from build123d import *

# Parameters (mm, degrees)
SKETCH1_W           = 22
SKETCH1_H           = 22
SKETCH1_W_2         = 20.1
SKETCH1_H_2         = 20.1
BOSS_EXTRUDE1_DEPTH = 15
SKETCH2_W           = 22
SKETCH2_H           = 22
BOSS_EXTRUDE2_DEPTH = 2


with BuildPart() as part:
    # Sketch1 → Boss-Extrude1 (new body)
    # profile 1 of 3: a face of its own
    with BuildSketch(Plane(origin=(0, 0, 0), x_dir=(1, 0, 0), z_dir=(0, 1, 0))):
        Rectangle(SKETCH1_W, SKETCH1_H)
        Rectangle(SKETCH1_W_2, SKETCH1_H_2, mode=Mode.SUBTRACT)
    # profile 2 of 3: a face of its own
    with BuildSketch(Plane(origin=(0, 0, 0), x_dir=(1, 0, 0), z_dir=(0, 1, 0))):
        Polygon((1.245, 10.05), (-1.245, 10.05), (-1.245, 8.05), (-5, 8.05), (-0.799132047, 5.15), (0.799132047, 5.15), (5, 8.05), (1.245, 8.05), align=None)
    # profile 3 of 3: a face of its own
    with BuildSketch(Plane(origin=(0, 0, 0), x_dir=(1, 0, 0), z_dir=(0, 1, 0))):
        Polygon((-1.245, -8.05), (-1.245, -10.05), (1.245, -10.05), (1.245, -8.05), (5, -8.05), (0.799132047, -5.15), (-0.799132047, -5.15), (-5, -8.05), align=None)
    extrude(amount=BOSS_EXTRUDE1_DEPTH)

    # Sketch2 → Boss-Extrude2 (add)
    with BuildSketch(Plane.XZ):
        Rectangle(SKETCH2_W, SKETCH2_H)
    extrude(amount=BOSS_EXTRUDE2_DEPTH)


solid = part.part
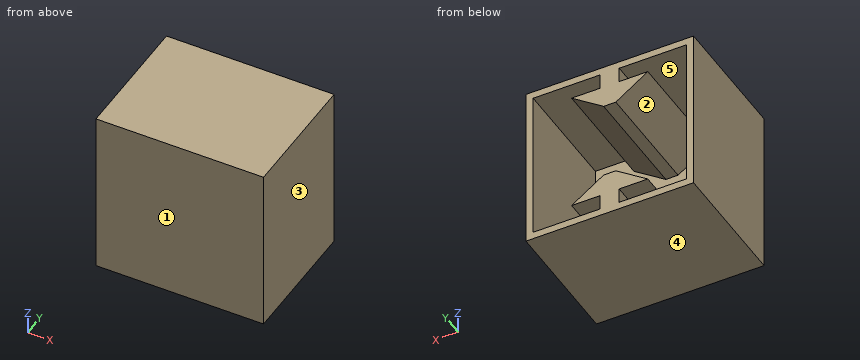
Model file for the job. Use its own axes, mm. Face numbers are marked on the shaded views. A direction names the side the tool comes from. Give positions to 0.01 mm unless a question says otherwise; leave off trailing zeros. Loops run counter-clockwise (first coordinate to the right, second up) from the corner with the lowest first, then second, coordinate; pieces in that order, holes last.
Item 1: Mould opens along X. For the marked faces 3, 4 and 5 say: +X half, -X half, draft (parallel to the pull), parting line (faces both ways), or undercut.
Check values:
face 3: +X half
face 4: draft
face 5: undercut
Item 2: Slice it at A-A (y = 6.5). Write the cut outline in (x, z) (3 decimals).
Check values:
outline: (-11, -11) - (11, -11) - (11, 11) - (-11, 11) - close; hole (-10.05, -10.05) - (-1.245, -10.05) - (-1.245, -8.05) - (-5, -8.05) - (-0.799, -5.15) - (0.799, -5.15) - (5, -8.05) - (1.245, -8.05) - (1.245, -10.05) - (10.05, -10.05) - (10.05, 10.05) - (1.245, 10.05) - (1.245, 8.05) - (5, 8.05) - (0.799, 5.15) - (-0.799, 5.15) - (-5, 8.05) - (-1.245, 8.05) - (-1.245, 10.05) - (-10.05, 10.05) - close
Item 3: Which spindle directions (+Z, -Z, +X, -X, +Y, -Y) get a long thin tool onto all of the face, cutting with end or side? Do the marked faces 1 and 2. Say none if no direction does.
Check values:
face 1: +Z, -Z, +X, -X, -Y
face 2: +Y
Item 4: Slice it at D-D (x = 4.5). Write the cut outline in (y, z).
Check values:
outline: (-2, -11) - (15, -11) - (15, -10.05) - (0, -10.05) - (0, -8.05) - (15, -8.05) - (15, -7.7) - (0, -7.7) - (0, 7.7) - (15, 7.7) - (15, 8.05) - (0, 8.05) - (0, 10.05) - (15, 10.05) - (15, 11) - (-2, 11) - close
Item 5: Slice it at C-C (z = -3.25). Write the cut outline in (x, y), plus the area to 3 significant figures.
Check values:
outline: (-11, -2) - (11, -2) - (11, 15) - (10.05, 15) - (10.05, 0) - (-10.05, 0) - (-10.05, 15) - (-11, 15) - close
area: 72.5 mm2
Item 6: Drill centre lines: line 1 along X through (y, z) = (9.5, 9) (3 decimals); line 2 along Z through (x, y) = (8, 4.25). Where is each one in solid material? Low to high.
Check values:
line 1: x = -11 to -10.05, -1.245 to 1.245, 10.05 to 11
line 2: z = -11 to -10.05, 10.05 to 11
Item 7: Drop a flat-ended pin along its axis: P1, Ø1.5, axis at x = 3.5, z = -1.5, coming from the +Y side. Give the stop position or say it passes through.
Check values:
P1: stops at y = 0
Item 8: Slice it at B-B (x = -8.5). Write the cut outline in (y, z), plus the area to 3 significant figures.
Check values:
outline: (-2, -11) - (15, -11) - (15, -10.05) - (0, -10.05) - (0, 10.05) - (15, 10.05) - (15, 11) - (-2, 11) - close
area: 72.5 mm2
